Here's how the part is built. I have some questions about the finished solid (model axes, mm). A direction names the side the tool comes from. Give positions to 0.01 mm unless a question says otherwise; leave off trailing zeros. Write each loop counter-clockwise with the first axis right and the second up, starting at its lowest first coordinate (ties: lowest second). Pieces come first, ordered by that corner, then holes. Notation, with made-up numbers: M 61,38.25 L 119,38.25 A14 ccw 119,55.25 Z; hole C -18,86 d4. An arc over 180 degrees is marked long. Answer as CSV lines item,"result". Start each with the question number.
Q1. If I drill on line 1 along X through (y, z) = (3.5, -0.4) (3 decimals); line 2 along Z through (x, y) = (-3.25, 2.8) (3 decimals); line 3 along X through (y, z) = (2.95, -0.6) (3 decimals), over which ranges is the centre line in solid material (lowest first)?
Q2. Suppose I cut it at B-B (y = 1.8). Count the separate pieces of the cut face and the enclosed holes in it, then the cut area to 3 significant figures.
Q3. Suppose I cut it at A-A (z = -0.7). Write out the boundary of the cut face in (x, y) (3 decimals), then the cut area to 3 significant figures.
Q4. Thinking about a two-plate mould opening in X: for faces 6 (the flat face through (-5, 2, -0.525)), 7 (the flat face through (-6.15, 2, 1)), 8 (the flat face through (-0.81, 2, 0)), which applies, +X half, -X half, draft (parallel to the pull), parting line (faces both ways), or undercut?
Q5. On a 3-axis mill with a long thin cutter (end or side, diameter ignored), from which of +Z, -Z, +X, -X, +Y, -Y can I reach the whole of each face in a straight line? I mean faces 1 (the flat face through (6.15, 2, 1)), 2 (the flat face through (-4.625, 2, -1)), 3 (the flat face through (1.73, 2, 0)), 4 (the flat face through (5, 2, -0.525)), 5 (the flat face through (0, 1, -1.725)). Say none if no direction works.
Q6. For pin 1 (0.5 mm diameter, centred on x = 5.5, y = 2.5, fed in from -Z) (3 decimals), with a flat end and sliding along its axis, tell me the tip position at first contact or that it passes through.
Q7. Suppose I cut it at C-C (x = 2.25). Write out the boundary of the cut face in (y, z) (3 decimals).
```python
from build123d import *

# Parameters (mm, degrees)
SKETCH1_W           = 1.525
SKETCH1_H           = 2.25
SKETCH1_W_2         = 9.25
SKETCH1_H_2         = 1.2
BOSS_EXTRUDE1_DEPTH = 4.2
SKETCH2_W           = 8.45
SKETCH2_H           = 2.65
CUT_EXTRUDE1_DEPTH  = 3.2
SKETCH3_W           = 8.45
SKETCH3_H           = 0.4
CUT_EXTRUDE2_DEPTH  = 1.6
SKETCH4_W           = 0.35
SKETCH4_H           = 1
BOSS_EXTRUDE2_DEPTH = 2.5


with BuildPart() as part:
    # Sketch1 → Boss-Extrude1 (new body)
    with BuildSketch(Plane(origin=(0, 0, 0), x_dir=(1, 0, 0), z_dir=(0, 1, 0))):
        with Locations((-5.3875, -0.6)):
            Rectangle(SKETCH1_W, SKETCH1_H)
        with Locations((0, 1.125)):
            Rectangle(SKETCH1_W_2, SKETCH1_H_2)
        with Locations((0, -0.6)):
            Rectangle(SKETCH1_W_2, SKETCH1_H)
        with Locations((5.3875, -0.6)):
            Rectangle(SKETCH1_W, SKETCH1_H)
    extrude(amount=BOSS_EXTRUDE1_DEPTH)

    # Sketch2 → Cut-Extrude1 (cut)
    with BuildSketch(Plane(origin=(0, 4.2, 0), x_dir=(1, 0, 0), z_dir=(0, 1, 0))):
        Rectangle(SKETCH2_W, SKETCH2_H)
    extrude(amount=-CUT_EXTRUDE1_DEPTH, mode=Mode.SUBTRACT)

    # Sketch3 → Cut-Extrude2 (cut)
    with BuildSketch(Plane(origin=(0, 4.2, 0), x_dir=(1, 0, 0), z_dir=(0, 1, 0))):
        with Locations((0, 1.525)):
            Rectangle(SKETCH3_W, SKETCH3_H)
    extrude(amount=-CUT_EXTRUDE2_DEPTH, mode=Mode.SUBTRACT)

    # Sketch4 → Boss-Extrude2 (add)
    with BuildSketch(Plane(origin=(0, 1, 0), x_dir=(1, 0, 0), z_dir=(0, 1, 0))):
        with Locations((0.635, -0.325)):
            Rectangle(SKETCH4_W, SKETCH4_H)
        with Locations((-0.635, -0.325)):
            Rectangle(SKETCH4_W, SKETCH4_H)
        with Locations((1.905, -0.325)):
            Rectangle(SKETCH4_W, SKETCH4_H)
        with Locations((3.175, -0.325)):
            Rectangle(SKETCH4_W, SKETCH4_H)
        with Locations((-3.175, -0.325)):
            Rectangle(SKETCH4_W, SKETCH4_H)
        with Locations((-1.905, -0.325)):
            Rectangle(SKETCH4_W, SKETCH4_H)
    extrude(amount=BOSS_EXTRUDE2_DEPTH)


solid = part.part
```
Resolved:
1,line 1,"-6.15 to -4.225, 4.225 to 6.15"
1,line 2,"-0.175 to 0.825, 1.325 to 1.725"
1,line 3,"-4.625 to -4.225, 4.225 to 4.625"
2,separate pieces,"7"
2,enclosed holes,"1"
2,area,"18.5 mm^2"
3,outline,"M -4.625,0 L 4.625,0 L 4.625,4.2 L 4.225,4.2 L 4.225,1 L -4.225,1 L -4.225,4.2 L -4.625,4.2 Z"
3,area,"11.8 mm^2"
4,face 6,"draft"
4,face 7,"-X half"
4,face 8,"undercut"
5,face 1,"+Z, -Z, +X, +Y, -Y"
5,face 2,"-Z, -X, +Y, -Y"
5,face 3,"+Y"
5,face 4,"-Z, +X, +Y, -Y"
5,face 5,"-Z, +X, -X, +Y, -Y"
6,pin 1,"z = -0.525"
7,outline,"M 0,-1.725 L 2.6,-1.725 L 2.6,-1.325 L 1,-1.325 L 1,1.325 L 4.2,1.325 L 4.2,1.725 L 0,1.725 Z"
